Part model, mm, in its own coordinate system. A direction names the side the tool comes from. Round coordinates to 2 decimals unless told otherwise and drop trailing zeros. Order: outer loops, then holes, each group sorted by start corner. A loop starts at its lowest first (then second) coordinate and runs counter-clockwise, first axis right, second up. Notation, with made-up numbers: (67, 17) - (98, 17) arc R12 ccw to (98, 22) - close; hole circle Ø3 at (85, 19.5). An arc over 180 degrees is marked (long way). Return JSON: item names as keys, results as strings. Group by question number.
Item 1: Drop flat-ended pins along their axis: pin 1 (1.3 mm diameter, centred on y = -21, z = 11, fed in from +X); pin 2 (3 mm diameter, centred on x = 29.5, y = -7.5, fed in from +Z). Give the stop position or say it passes through.
Item 2: Saw through at A-A on z = 6.35. List the corners of the cut face in (x, y), and give its area (3 significant figures).
Item 3: Probe probe 1 along Y at (x, z) = (0, 4.25); probe 2 along X at (y, z) = (0.5, 6.5); probe 3 along X at (y, z) = (5, 11). List the from-to ranges inside material, lowest first.
Item 4: Saw through at C-C on x = 9.5. List the corners of the cut face in (y, z), and give its area (3 significant figures).
Item 5: Saw through at D-D on y = 0. List the corners of the cut face in (x, z).
Item 6: Tool access for faces 4 (the face through (32.781, -0.356, 10.124)), 5 (the face through (-29.21, 0, 11)), 6 (the face through (-1, 25.4, 6)): list every direction of +Z, -Z, +X, -X, +Y, -Y with a clear straight run to the whole face (end or side of a thin tool).
Item 7: Two-plate mould, pull along Y, no slides. Class faces 1 (the face through (-1, -25.4, 6)), 2 (the face through (-18, 0, 12.7)), 3 (the face through (12.114, 3.815, 6.261)): released by +Y, released by -Y, zero draft, split by the parting line, or undercut.
Item 8: Saw through at B-B on y = 20.5. List the corners of the cut face in (x, z), and give its area (3 significant figures).
```python
from build123d import *

# Parameters (mm, degrees)
F0_W     = 76.2
F0_H     = 50.8
F0_R     = 12.7
F1_DEPTH = 12.7
F2_W     = 6.35
F2_H     = 50.8
F3_DEPTH = 2.54
F5_DEPTH = 50.801
F6_R     = 4.7625
F7_DEPTH = 12.7


with BuildPart() as f1:
    # F0 (on Top) → F1 (new body)
    with BuildSketch(Plane.XY):
        Rectangle(F0_W, F0_H)
        Circle(F0_R, mode=Mode.SUBTRACT)
    extrude(amount=F1_DEPTH)

    # F2 (on face) → F3 (cut)
    with BuildSketch(Plane.XY.offset(12.7)):
        with BuildLine():
            ThreePointArc((4.624233052, 11.8282064862), (-0.4973552707, 12.6902575913), (-5.535766948, 11.4300168109))
            Line((-5.535766948, 11.4300168109), (-5.535766948, -11.4300168109))
            ThreePointArc((-5.535766948, -11.4300168109), (-0.4973552707, -12.6902575913), (4.624233052, -11.8282064862))
            Line((4.624233052, -11.8282064862), (4.624233052, 11.8282064862))
        make_face()
        with Locations((-32.385, 0)):
            Rectangle(F2_W, F2_H)
        with BuildLine():
            Line((-5.535766948, -11.4300168109), (-5.535766948, -25.4))
            Line((-5.535766948, -25.4), (4.624233052, -25.4))
            Line((4.624233052, -25.4), (4.624233052, -11.8282064862))
            ThreePointArc((4.624233052, -11.8282064862), (-0.4973552707, -12.6902575913), (-5.535766948, -11.4300168109))
        make_face()
        with BuildLine():
            Line((4.624233052, 25.4), (-5.535766948, 25.4))
            Line((-5.535766948, 25.4), (-5.535766948, 11.4300168109))
            ThreePointArc((-5.535766948, 11.4300168109), (-0.4973552707, 12.6902575913), (4.624233052, 11.8282064862))
            Line((4.624233052, 11.8282064862), (4.624233052, 25.4))
        make_face()
    extrude(amount=-F3_DEPTH, mode=Mode.SUBTRACT)

    # F4 (on face) → F5 (cut, through all)
    with BuildSketch(Plane.XZ.offset(25.4)):
        Polygon((31.294233052, 12.7), (18.594233052, 12.7), (15.6612936845, 7.62), (34.2271724195, 7.62), align=None)
    extrude(amount=-F5_DEPTH, mode=Mode.SUBTRACT)

    # F6 (on face) → F7 (join)
    with BuildSketch(Plane.YZ.offset(38.1)):
        with Locations((0, 6.35)):
            Circle(F6_R)
    extrude(amount=F7_DEPTH)


solid = f1.part
```
Filled in:
{
 "1": {"pin 1": "stops at x = 38.1", "pin 2": "stops at z = 7.62"},
 "2": {"outline": "(-38.1, -25.4) - (38.1, -25.4) - (38.1, -4.76) - (50.8, -4.76) - (50.8, 4.76) - (38.1, 4.76) - (38.1, 25.4) - (-38.1, 25.4) - close; hole circle Ø25.4 at (0, 0)", "area": "3,490 mm^2"},
 "3": {"probe 1": "y = -25.4 to -12.7, 12.7 to 25.4", "probe 2": "x = -38.1 to -12.69, 12.69 to 50.8", "probe 3": "x = -38.1 to -35.56, -29.21 to -11.67, 11.67 to 17.61, 32.28 to 38.1"},
 "4": {"outline": "(-25.4, 0) - (-8.43, 0) - (-8.43, 12.7) - (-25.4, 12.7) - close; (8.43, 0) - (25.4, 0) - (25.4, 12.7) - (8.43, 12.7) - close", "area": "431 mm^2"},
 "5": {"outline": "(-38.1, 0) - (-12.7, 0) - (-12.7, 12.7) - (-29.21, 12.7) - (-29.21, 10.16) - (-35.56, 10.16) - (-35.56, 12.7) - (-38.1, 12.7) - close; (12.7, 0) - (38.1, 0) - (38.1, 1.59) - (50.8, 1.59) - (50.8, 11.11) - (38.1, 11.11) - (38.1, 12.7) - (31.29, 12.7) - (34.23, 7.62) - (15.66, 7.62) - (18.59, 12.7) - (12.7, 12.7) - close"},
 "6": {"face 4": "+Y, -Y", "face 5": "+Z, +Y, -Y", "face 6": "+Z, -Z, +X, -X, +Y"},
 "7": {"face 1": "released by -Y", "face 2": "zero draft", "face 3": "undercut"},
 "8": {"outline": "(-38.1, 0) - (38.1, 0) - (38.1, 12.7) - (31.29, 12.7) - (34.23, 7.62) - (15.66, 7.62) - (18.59, 12.7) - (4.62, 12.7) - (4.62, 10.16) - (-5.54, 10.16) - (-5.54, 12.7) - (-29.21, 12.7) - (-29.21, 10.16) - (-35.56, 10.16) - (-35.56, 12.7) - (-38.1, 12.7) - close", "area": "846 mm^2"}
}
